Check sheet for the modelled part. Datum: model origin and axes. Units: mm. Face numbers are marked on the shaded views. A direction names the side the tool comes from. Coordinates: 2 decimals unless noted, no trailing zeros. Loops run counter-clockwise (first coordinate to the right, second up) from the corner with the lowest first, then second, coordinate; pieces in that order, holes last.
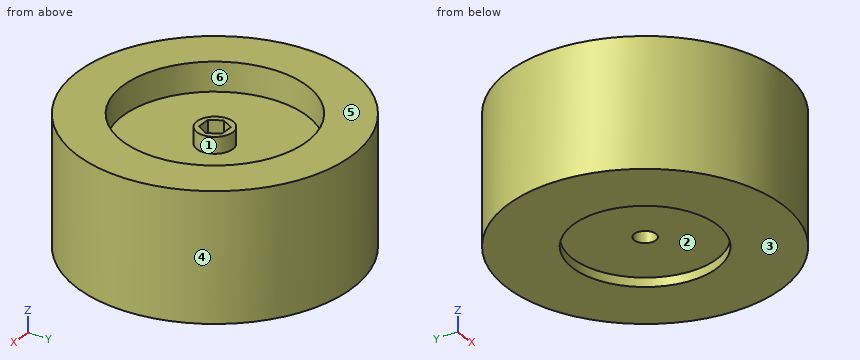
```python
from build123d import *

# Parameters (mm, degrees)
SKETCH2_R                      = 48.5
BOSS_EXTRUDE1_DEPTH            = 22.45
SKETCH3_R                      = 32.5
CUT_EXTRUDE1_DEPTH             = 10.16
SKETCH9_R                      = 6.35
BOSS_EXTRUDE2_DEPTH            = 5.715
CUT_EXTRUDE2_DEPTH             = 77.885418644
CUT_EXTRUDE2_DEPTH_BACK        = 22.1
M5_CLEARANCE_HOLE1_D           = 5.5
M5_CLEARANCE_HOLE1_CSINK_D     = 5.55
M5_CLEARANCE_HOLE1_CSINK_ANGLE = 90
SKETCH8_R                      = 3.81
CUT_EXTRUDE3_DEPTH             = 8.255
SKETCH10_R                     = 25.4
CUT_EXTRUDE4_DEPTH             = 3.175


with BuildPart() as part:
    # Sketch2 → Boss-Extrude1 (new, symmetric)
    with BuildSketch(Plane.XY):
        Circle(SKETCH2_R)
    extrude(amount=BOSS_EXTRUDE1_DEPTH, both=True)

    # Sketch3 → Cut-Extrude1 (cut)
    with BuildSketch(Plane.XY.offset(22.45)):
        Circle(SKETCH3_R)
    extrude(amount=-CUT_EXTRUDE1_DEPTH, mode=Mode.SUBTRACT)

    # Sketch9 → Boss-Extrude2 (add)
    with BuildSketch(Plane.XY.offset(12.29)):
        Circle(SKETCH9_R)
    extrude(amount=BOSS_EXTRUDE2_DEPTH)

    # Sketch4 → Cut-Extrude2 (cut, two sides: drawn at the far end of the back side and taken through both)
    with BuildSketch(Plane.XY.offset(12.29).offset(-CUT_EXTRUDE2_DEPTH_BACK)):
        Polygon((2.38156986, 4.125), (-2.38156986, 4.125), (-4.763139721, 0), (-2.38156986, -4.125), (2.38156986, -4.125), (4.763139721, 0), align=None)
    extrude(amount=CUT_EXTRUDE2_DEPTH + CUT_EXTRUDE2_DEPTH_BACK, mode=Mode.SUBTRACT)

    # M5 Clearance Hole1 (through all)
    with Locations(Plane.XY.offset(-9.81)):
        with Locations((0, 0)):
            CounterSinkHole(M5_CLEARANCE_HOLE1_D / 2, M5_CLEARANCE_HOLE1_CSINK_D / 2, counter_sink_angle=M5_CLEARANCE_HOLE1_CSINK_ANGLE)

    # Sketch8 → Cut-Extrude3 (cut)
    with BuildSketch(Plane(origin=(0, 0, -22.45), x_dir=(-1, 0, 0), z_dir=(0, 0, -1))):
        Circle(SKETCH8_R)
    extrude(amount=-CUT_EXTRUDE3_DEPTH, mode=Mode.SUBTRACT)

    # Sketch10 → Cut-Extrude4 (cut)
    with BuildSketch(Plane(origin=(0, 0, -22.45), x_dir=(-1, 0, 0), z_dir=(0, 0, -1))):
        Circle(SKETCH10_R)
    extrude(amount=-CUT_EXTRUDE4_DEPTH, mode=Mode.SUBTRACT)


solid = part.part
```
1) Section check D-D on x = 18. Enter the section's corners in (y, z) (3 decimals), plus the area to 3 significant figures.
Answer sheet:
outline: (-45.036, -22.45) - (-17.921, -22.45) - (-17.921, -19.275) - (17.921, -19.275) - (17.921, -22.45) - (45.036, -22.45) - (45.036, 22.45) - (27.06, 22.45) - (27.06, 12.29) - (-27.06, 12.29) - (-27.06, 22.45) - (-45.036, 22.45) - close
area: 3,380 mm2
2) Depth check by flat-ended pin: pin 1 (4 mm diameter, centred on x = -35.5, z = -11, fed in from +Y); pin 2 (3 mm diameter, centred on y = -19, z = 11.5, fed in from +X); pin 3 (12 mm diameter, centred on x = 0, y = 0, fed in from -Z) (3 decimals). Enter the tip coordinate at first touch or a pass-through.
Answer sheet:
pin 1: stops at y = 35.07
pin 2: stops at x = 45.23
pin 3: stops at z = -19.275
3) Scan lines: line 1 (Y direction, x = 1, z = -5.5) (3 decimals); line 2 (Z direction, x = -0.5, y = 12.5) (3 decimals); line 3 (Y direction, x = 0, z = -16). Record each from-to range of solid material in increasing order.
Answer sheet:
line 1: y = -48.49 to -4.125, 4.125 to 48.49
line 2: z = -19.275 to 12.29
line 3: y = -48.5 to -3.81, 3.81 to 48.5
4) Section check B-B on z = 5. Enter the section's corners in (x, y) (3 decimals), plus the area to 3 significant figures.
Answer sheet:
outline: circle Ø97 at (0, 0); hole (-4.763, 0) - (-2.382, -4.125) - (2.382, -4.125) - (4.763, 0) - (2.382, 4.125) - (-2.382, 4.125) - close
area: 7,330 mm2
5) Set-up check for the marked faces 1, 2 and 3: record each of +Z, -Z, +X, -X, +Y, -Y from which the full face is reachable in a straight line by a thin tool's end or side.
Answer sheet:
face 1: +Z
face 2: -Z
face 3: -Z, +X, -X, +Y, -Y
6) Section check C-C on y = 8. Enter the section's corners in (x, z) (3 decimals).
Answer sheet:
outline: (-47.836, -22.45) - (-24.107, -22.45) - (-24.107, -19.275) - (24.107, -19.275) - (24.107, -22.45) - (47.836, -22.45) - (47.836, 22.45) - (31.5, 22.45) - (31.5, 12.29) - (-31.5, 12.29) - (-31.5, 22.45) - (-47.836, 22.45) - close
7) Mould release check, pull along Y, two halves, no side actions. Record for the marked faces 4, 5 and 6: +Y half, -Y half, draft (parallel to the pull), parting line (faces both ways), or undercut.
Answer sheet:
face 4: parting line
face 5: draft
face 6: undercut
